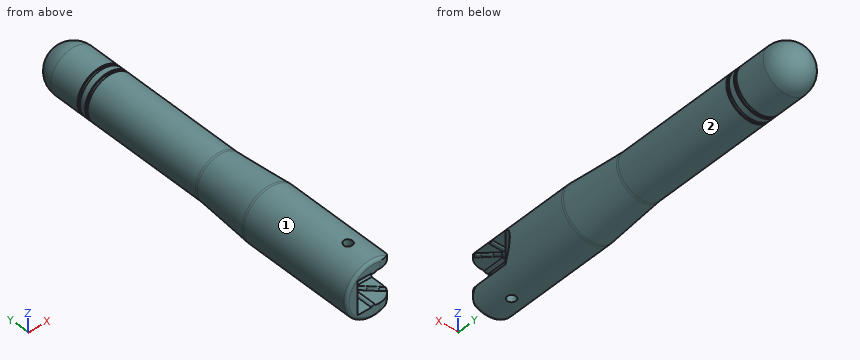
```python
from build123d import *

# Parameters (mm, degrees)
ESQUISSE3_W                  = 7.5
ESQUISSE3_H                  = 5.8
ENL_V_MAT_EXTRU_1_DEPTH      = 8
CONG_1_R                     = 0.5
ENL_V_MAT_EXTRU_2_DEPTH      = 64.516622885
ENL_V_MAT_EXTRU_2_DEPTH_BACK = 64.516622885
ESQUISSE4_R                  = 0.75
ESQUISSE5_W                  = 0.75
ESQUISSE5_H                  = 3.75
ESQUISSE5_W_2                = 2.511980861
ESQUISSE5_H_2                = 0.75
BOSS_EXTRU_1_DEPTH           = 0.2
CONG_2_R                     = 0.2
CONG_2_OF_SYM_TRIE1_R        = 0.2
ENL_V_MAT_EXTRU_3_DEPTH      = 64.799070395


with BuildPart() as part:
    # Esquisse2 → Révolution1 (revolve)
    with BuildSketch(Plane.XY):
        with BuildLine():
            Line((4.014003451, 30.213287326), (4.735996549, 20.586712674))
            ThreePointArc((4.735996549, 20.586712674), (4.746497911, 20.399868856), (4.75, 20.212762933))
            Line((4.75, 20.212762933), (4.75, 0))
            Line((4.75, 0), (1, 0))
            Line((1, 0), (1, 59.160402))
            Line((1, 59.160402), (0, 59.160402))
            Line((0, 59.160402), (0, 63.160402))
            ThreePointArc((0, 63.160402), (2.828427125, 61.988829125), (4, 59.160402))
            Line((4, 59.160402), (4, 53.860402))
            Line((4, 53.860402), (3.75, 53.860402))
            Line((3.75, 53.860402), (3.75, 53.360402))
            Line((3.75, 53.360402), (4, 53.360402))
            Line((4, 53.360402), (4, 52.360402))
            Line((4, 52.360402), (3.75, 52.360402))
            Line((3.75, 52.360402), (3.75, 51.860402))
            Line((3.75, 51.860402), (4, 51.860402))
            Line((4, 51.860402), (4, 30.587237067))
            ThreePointArc((4, 30.587237067), (4.003502089, 30.400131144), (4.014003451, 30.213287326))
        make_face()
    revolve(axis=Axis((0, 0, 0), (0, 1, 0)))

    # Esquisse3 → Enlèv. mat.-Extru.1 (cut)
    with BuildSketch(Plane.XZ):
        with Locations((1, 0)):
            Rectangle(ESQUISSE3_W, ESQUISSE3_H)
    extrude(amount=-ENL_V_MAT_EXTRU_1_DEPTH, mode=Mode.SUBTRACT)

    # Congé1
    cong_1_edges = [part.edges().sort_by_distance(p)[0] for p in [
        (-4.75, 0, 0),
    ]]
    fillet(cong_1_edges, radius=CONG_1_R)

    # Esquisse4 → Enlèv. mat.-Extru.2 (cut, two sides: drawn at the far end of the back side and taken through both)
    with BuildSketch(Plane.XY.offset(-ENL_V_MAT_EXTRU_2_DEPTH_BACK)):
        with Locations((0, 5)):
            Circle(ESQUISSE4_R)
        with BuildLine():
            Line((1.161980861, 0), (3.761980861, 0))
            Line((3.761980861, 0), (3.761980861, 2.6))
            ThreePointArc((3.761980861, 2.6), (3.000458492, 0.761522369), (1.161980861, 0))
        make_face()
        Polygon((3.761980861, 8), (4.75, 10), (4.75, 8), align=None)
    extrude(amount=ENL_V_MAT_EXTRU_2_DEPTH + ENL_V_MAT_EXTRU_2_DEPTH_BACK, mode=Mode.SUBTRACT)

    # Esquisse5 → Boss.-Extru.1 (add)
    with BuildSketch(Plane.XY.offset(-2.9)):
        with Locations((0, 1.875)):
            Rectangle(ESQUISSE5_W, ESQUISSE5_H)
        Polygon((0.618718434, 3.850951481), (1.149048519, 4.381281566), (4.027145904, 1.503184182), (3.496815818, 0.972854096), align=None)
        with Locations((2.50599043, 5)):
            Rectangle(ESQUISSE5_W_2, ESQUISSE5_H_2)
    boss_extru_1 = extrude(amount=BOSS_EXTRU_1_DEPTH)

    # Congé2
    cong_2_edges = [part.edges().sort_by_distance(p)[0] for p in [
        (2.505990431, 5.375, -2.7),
        (2.505990431, 4.625, -2.7),
        (2.588097212, 2.942232874, -2.7),
        (2.057767126, 2.411902788, -2.7),
        (-0.375, 1.875, -2.7),
        (0.375, 1.875, -2.7),
    ]]
    fillet(cong_2_edges, radius=CONG_2_R - 0.0001)  # a hair under: the kernel refuses the full size

    # Symétrie1: Boss.-Extru.1 across plane
    add(boss_extru_1.mirror(Plane.XY))

    # Congé2 of Symétrie1
    cong_2_of_sym_trie1_edges = [part.edges().sort_by_distance(p)[0] for p in [
        (2.505990431, 5.375, 2.7),
        (2.505990431, 4.625, 2.7),
        (2.588097212, 2.942232874, 2.7),
        (2.057767126, 2.411902788, 2.7),
        (-0.375, 1.875, 2.7),
        (0.375, 1.875, 2.7),
    ]]
    fillet(cong_2_of_sym_trie1_edges, radius=CONG_2_OF_SYM_TRIE1_R - 0.0001)  # a hair under: the kernel refuses the full size

    # Esquisse6 → Enlèv. mat.-Extru.3 (cut, through all)
    with BuildSketch(Plane.XY.offset(2.9)):
        with BuildLine():
            Line((4.027145904, 1.503184182), (3.658059706, 1.87227038))
            ThreePointArc((3.658059706, 1.87227038), (3.516870908, 1.49795968), (3.319930166, 1.149739748))
            Line((3.319930166, 1.149739748), (3.496815818, 0.972854096))
            Line((3.496815818, 0.972854096), (4.027145904, 1.503184182))
        make_face()
    extrude(amount=-ENL_V_MAT_EXTRU_3_DEPTH, mode=Mode.SUBTRACT)


solid = part.part
```
Part model, mm, in its own coordinate system. Face numbers are marked on the shaded views. A direction names the side the tool comes from. Round coordinates to 2 decimals unless told otherwise and drop trailing zeros. Write each loop counter-clockwise with the first axis right and the second up, starting at its lowest first coordinate (ties: lowest second). Pieces come first, ordered by that corner, then holes.
Item 1: Probe L1, parallel to X at y = 5, z = 3.9; L2, parallel to Z at x = 0, y = 38.5; L3, parallel to X at y = 12, z = 0.5. List the from-to ranges inside material, lowest first.
Results:
L1: x = -2.71 to -0.75, 0.75 to 2.71
L2: z = -4 to -1, 1 to 4
L3: x = -4.72 to -0.87, 0.87 to 4.72
Item 2: Cut at A-A, the plane y = 42. Give the cut face in (x, z).
Results:
outline: circle Ø8 at (0, 0); hole circle Ø2 at (0, 0)
Item 3: Cut at B-B, the plane y = 26. Give the cut face in (x, z), plus the area to 3 significant figures.
Results:
outline: circle Ø8.66 at (0, 0); hole circle Ø2 at (0, 0)
area: 55.8 mm2
Item 4: Which spindle directions (+Z, -Z, +X, -X, +Y, -Y) get a long thin tool onto all of the face, cutting with end or side? Do the marked faces 1 and 2. Say none if no direction does.
Results:
face 1: +Y, -Y
face 2: +Y
Item 5: Drop flat-ended pins along their axis: pin 1 Ø2.5 at (x, z) = (-0.5, -2) entering from +Y; pin 2 Ø2.5 at (x, z) = (2, -0.5) entering from -Y; pin 3 Ø4 at (x, y) = (-0.5, 17.5) entering from +Z; pin 4 Ø1.5 at (y, z) = (20.5, 4) entering from +X. Give the stop position or say it passes through.
Results:
pin 1: stops at y = 63.08
pin 2: stops at y = 8
pin 3: stops at z = 4.75
pin 4: stops at x = 3.45
